from build123d import *

# Parameters (mm, degrees)
F0_W     = 3
F0_H     = 3
F1_DEPTH = 2
F2_R     = 1.5
F3_DEPTH = 2.001


with BuildPart() as f1:
    # F0 (on Top) → F1 (new body)
    with BuildSketch(Plane.XY):
        with BuildLine():
            ThreePointArc((-1.9371370628, -1.5), (-2.45, 0), (-1.9371370628, 1.5))
            Line((-1.9371370628, 1.5), (-7.5, 1.5))
            Line((-7.5, 1.5), (-7.5, -1.5))
            Line((-7.5, -1.5), (-1.9371370628, -1.5))
        make_face()
        Rectangle(F0_W, F0_H)
        with BuildLine():
            Line((-1.5, -1.5), (-1.5, 1.5))
            Line((-1.5, 1.5), (-1.9371370628, 1.5))
            ThreePointArc((-1.9371370628, 1.5), (-2.45, 0), (-1.9371370628, -1.5))
            Line((-1.9371370628, -1.5), (-1.5, -1.5))
        make_face()
        with BuildLine():
            ThreePointArc((1.9371370628, 1.5), (2.3182413381, 0.7926267079), (2.45, 0))
            ThreePointArc((2.45, 0), (2.3182413381, -0.7926267079), (1.9371370628, -1.5))
            Line((1.9371370628, -1.5), (7.5, -1.5))
            Line((7.5, -1.5), (7.5, 1.5))
            Line((7.5, 1.5), (1.9371370628, 1.5))
        make_face()
        with BuildLine():
            Line((1.5, -7.5), (1.5, -1.9371370628))
            ThreePointArc((1.5, -1.9371370628), (0, -2.45), (-1.5, -1.9371370628))
            Line((-1.5, -1.9371370628), (-1.5, -7.5))
            Line((-1.5, -7.5), (1.5, -7.5))
        make_face()
        with BuildLine():
            Line((1.5, 1.5), (1.5, 1.9371370628))
            ThreePointArc((1.5, 1.9371370628), (0, 2.45), (-1.5, 1.9371370628))
            Line((-1.5, 1.9371370628), (-1.5, 1.5))
            Line((-1.5, 1.5), (1.5, 1.5))
        make_face()
        with BuildLine():
            ThreePointArc((1.9371370628, -1.5), (2.3182413381, -0.7926267079), (2.45, 0))
            ThreePointArc((2.45, 0), (2.3182413381, 0.7926267079), (1.9371370628, 1.5))
            Line((1.9371370628, 1.5), (1.5, 1.5))
            Line((1.5, 1.5), (1.5, -1.5))
            Line((1.5, -1.5), (1.9371370628, -1.5))
        make_face()
        with BuildLine():
            ThreePointArc((-1.5, 1.9371370628), (0, 2.45), (1.5, 1.9371370628))
            Line((1.5, 1.9371370628), (1.5, 7.5))
            Line((1.5, 7.5), (-1.5, 7.5))
            Line((-1.5, 7.5), (-1.5, 1.9371370628))
        make_face()
        with BuildLine():
            ThreePointArc((-1.5, -1.9371370628), (0, -2.45), (1.5, -1.9371370628))
            Line((1.5, -1.9371370628), (1.5, -1.5))
            Line((1.5, -1.5), (-1.5, -1.5))
            Line((-1.5, -1.5), (-1.5, -1.9371370628))
        make_face()
        with BuildLine():
            ThreePointArc((-1.9371370628, -1.5), (-1.7324116139, -1.7324116139), (-1.5, -1.9371370628))
            Line((-1.5, -1.9371370628), (-1.5, -1.5))
            Line((-1.5, -1.5), (-1.9371370628, -1.5))
        make_face()
        with BuildLine():
            Line((1.5, 1.5), (1.9371370628, 1.5))
            ThreePointArc((1.9371370628, 1.5), (1.7324116139, 1.7324116139), (1.5, 1.9371370628))
            Line((1.5, 1.9371370628), (1.5, 1.5))
        make_face()
        with BuildLine():
            ThreePointArc((1.5, -1.9371370628), (1.7324116139, -1.7324116139), (1.9371370628, -1.5))
            Line((1.9371370628, -1.5), (1.5, -1.5))
            Line((1.5, -1.5), (1.5, -1.9371370628))
        make_face()
        with BuildLine():
            Line((-1.5, 1.5), (-1.5, 1.9371370628))
            ThreePointArc((-1.5, 1.9371370628), (-1.7324116139, 1.7324116139), (-1.9371370628, 1.5))
            Line((-1.9371370628, 1.5), (-1.5, 1.5))
        make_face()
    extrude(amount=F1_DEPTH)

    # F2 (on face) → F3 (cut, through all)
    with BuildSketch(Plane.XY.offset(2)):
        Circle(F2_R)
    extrude(amount=-F3_DEPTH, mode=Mode.SUBTRACT)


solid = f1.part
The model under review builds one solid part; all positions refer to its coordinate system, in mm. A direction names the side the tool comes from. Give positions to 0.01 mm unless a question says otherwise; leave off trailing zeros. Write each loop counter-clockwise with the first axis right and the second up, starting at its lowest first coordinate (ties: lowest second). Pieces come first, ordered by that corner, then holes.
1. Add section B-B, the plane y = 0. Write out the cut boundary in (x, z), plus the area to 3 significant figures.
2. For P1, Ø1, axis at y = -4.5, z = 1.5, coming from the -X side; P2, Ø0.6, axis at y = -4, z = 1.5, coming from the +X side; P3, Ø1, axis at x = -4.5, z = 1, coming from the +Y side; P4, Ø6, axis at x = -3.5, y = 4.5, coming from the -Z side, all flat-tipped, find the tip position at first contact; note any pin that passes through.
3. Add section A-A, the plane z = 1.25. Write out the cut boundary in (x, y), plus the area to 3 significant figures.
4. Add section D-D, the plane y = -5.25. Write out the cut boundary in (x, z), plus the area to 3 significant figures.
5. Draft analysis for pull direction Y (two halves, no side actions). For faces 1 (the flat face through (0, 7.5, 1)), 2 (the flat face through (1.5, 5, 1)), 3 (the cylindrical face through (-1.5, 0.07, 1.01)), 4 (the flat face through (0, -7.5, 1)), state which applies: +Y half, -Y half, draft (parallel to the pull), parting line (faces both ways), or undercut.
6. Wall thickness on L1, parallel to Y at x = 0, z = 0.9; L2, parallel to X at y = 4.5, z = 1.6: over which ranges is each line inside the solid? List them lowest first.
7. Tool access review of faces 5 (the flat face through (-1.5, -5, 1)), 6 (the flat face through (5, 1.5, 1)), 7 (the flat face through (-2, 0, 0)), 8 (the flat face through (-1.5, 5, 1)), 9 (the flat face through (1.5, -5, 1)): name each direction out of +Z, -Z, +X, -X, +Y, -Y from which nothing blocks a thin tool from reaching the whole face with its end or side.
Worked answers:
1. outline: (-7.5, 0) - (-1.5, 0) - (-1.5, 2) - (-7.5, 2) - close; (1.5, 0) - (7.5, 0) - (7.5, 2) - (1.5, 2) - close
1. area: 24.0 mm2
2. P1: stops at x = -1.5
2. P2: stops at x = 1.5
2. P3: stops at y = 1.5
2. P4: stops at z = 0
3. outline: (-7.5, -1.5) - (-1.94, -1.5) arc R2.45 ccw to (-1.5, -1.94) - (-1.5, -7.5) - (1.5, -7.5) - (1.5, -1.94) arc R2.45 ccw to (1.94, -1.5) - (7.5, -1.5) - (7.5, 1.5) - (1.94, 1.5) arc R2.45 ccw to (1.5, 1.94) - (1.5, 7.5) - (-1.5, 7.5) - (-1.5, 1.94) arc R2.45 ccw to (-1.94, 1.5) - (-7.5, 1.5) - close; hole circle Ø3 at (0, 0)
3. area: 74.3 mm2
4. outline: (-1.5, 0) - (1.5, 0) - (1.5, 2) - (-1.5, 2) - close
4. area: 6.00 mm2
5. face 1: +Y half
5. face 2: draft
5. face 3: undercut
5. face 4: -Y half
6. L1: y = -7.5 to -1.5, 1.5 to 7.5
6. L2: x = -1.5 to 1.5
7. face 5: +Z, -Z, -X, -Y
7. face 6: +Z, -Z, +X, +Y
7. face 7: -Z, +X, -X, +Y, -Y
7. face 8: +Z, -Z, -X, +Y
7. face 9: +Z, -Z, +X, -Y
